For this review, take the finished solid that the model builds, in its own axes (mm). Face numbers are marked on the shaded views. A direction names the side the tool comes from. Give positions to 0.01 mm unless a question says otherwise; leave off trailing zeros. Order: outer loops, then holes, each group sorted by start corner. A loop starts at its lowest first (then second) coordinate and runs counter-clockwise, first axis right, second up. Notation, with made-up numbers: M -38.75,69.25 L -31.75,69.25 A28 cw -31.75,103.25 Z; hole C -1.75,71 d3. An arc over 180 degrees is marked long. Answer as CSV lines item,"result". Start each with the question number.
1. Mouldability with a two-part tool opening along X and no side actions: class the marked faces 1, 2 and 3 as pulls with the +X half, pulls with the -X half, needs draft (parallel to the pull), parting line crosses it, or undercut.
2. We need section D-D, the plane z = 9. Give the boundary of the cut face in (x, y), and give its area (3 significant figures).
3. We need section C-C, the plane x = 7.5. Give the boundary of the cut face in (y, z), and give its area (3 significant figures).
4. Clearance check with flat-ended pins moving along their axes: P1, Ø2.5, axis at x = 7.5, z = 12.5, coming from the +Y side; P2, Ø5, axis at x = 2.5, y = 58, coming from the +Z side. State where each tip first meets the part, or that it passes through.
5. For line 1 along Y through (x, z) = (7.5, 2.8); line 2 along Y through (x, z) = (9.5, 6); line 3 along X through (y, z) = (57.5, 7.25), list the stretches that pass through material, from the lowest coordinate up.
6. Machinability: for the marked faces 4 and 5, which of the approach directions +Z, -Z, +X, -X, +Y, -Y give a long, thin tool a straight path to every point of the face, cutting with its end or side? Answer none if there is none.
7. We need section B-B, the plane z = 12.5. Give the boundary of the cut face in (x, y), and give its area (3 significant figures).
8. We need section A-A, the plane y = 35. Give the boundary of the cut face in (x, z).
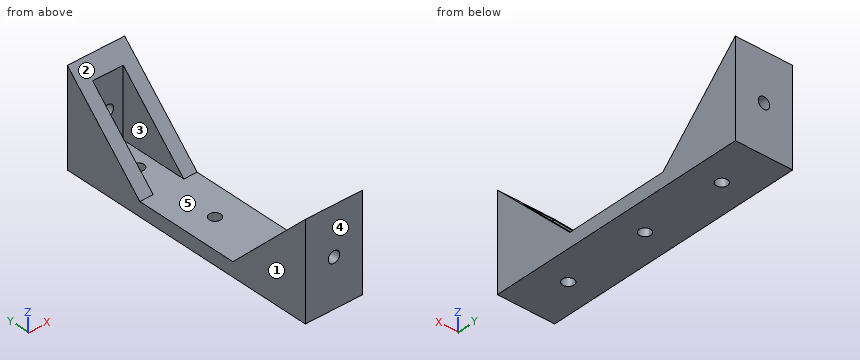
from build123d import *

# Parameters (mm, degrees)
F0_W     = 15
F0_H     = 70
F1_DEPTH = 25
F3_DEPTH = 25
F5_DEPTH = 25
F6_R     = 1.5
F7_DEPTH = 83.8
F8_R     = 1.5
F9_DEPTH = 25


with BuildPart() as f1:
    # F0 (on Top) → F1 (new body)
    with BuildSketch(Plane.XY):
        with Locations((7.5, 35)):
            Rectangle(F0_W, F0_H)
    extrude(amount=F1_DEPTH)

    # F2 (on face) → F3 (cut)
    with BuildSketch(Plane(origin=(0, 0, 0), x_dir=(0, -1, 0), z_dir=(-1, 0, 0))):
        Polygon((-35, 25), (-70, 25), (-48.676951, 3.676951), (-35, 3.676951), (-21.323049, 3.676951), (0, 25), align=None)
    extrude(amount=-F3_DEPTH, mode=Mode.SUBTRACT)

    # F4 (on face) → F5 (cut)
    with BuildSketch(Plane.XY.offset(3.676951)):
        Polygon((3.5, 66.5), (3.5, 35), (3.5, 3.5), (11.5, 3.5), (11.5, 35), (11.5, 66.5), align=None)
    extrude(amount=F5_DEPTH, mode=Mode.SUBTRACT)

    # F6 (on face) → F7 (cut)
    with BuildSketch(Plane.XZ):
        with Locations((7.5, 12.5)):
            Circle(F6_R)
    extrude(amount=-F7_DEPTH, mode=Mode.SUBTRACT)

    # F8 (on face) → F9 (cut)
    with BuildSketch(Plane.XY.offset(3.676951)):
        with Locations((7.5, 57.588476)):
            Circle(F8_R)
        with Locations((7.5, 12.411524)):
            Circle(F8_R)
        with Locations((7.5, 35)):
            Circle(F8_R)
    extrude(amount=-F9_DEPTH, mode=Mode.SUBTRACT)


solid = f1.part
Result set:
1,face 1,"pulls with the -X half"
1,face 2,"needs draft"
1,face 3,"undercut"
2,outline,"M 0,0 L 15,0 L 15,16 L 11.5,16 L 11.5,3.5 L 3.5,3.5 L 3.5,16 L 0,16 Z; M 0,54 L 3.5,54 L 3.5,66.5 L 11.5,66.5 L 11.5,54 L 15,54 L 15,70 L 0,70 Z"
2,area,"280 mm2"
3,outline,"M 0,0 L 10.91,0 L 10.91,3.68 L 3.5,3.68 L 3.5,11 L 0,11 Z; M 0,14 L 3.5,14 L 3.5,21.5 L 0,25 Z; M 13.91,0 L 33.5,0 L 33.5,3.68 L 13.91,3.68 Z; M 36.5,0 L 56.09,0 L 56.09,3.68 L 36.5,3.68 Z; M 59.09,0 L 70,0 L 70,11 L 66.5,11 L 66.5,3.68 L 59.09,3.68 Z; M 66.5,14 L 70,14 L 70,25 L 66.5,21.5 Z"
3,area,"340 mm2"
4,P1,"through"
4,P2,"z = 15.5"
5,line 1,"0 to 10.91, 13.91 to 33.5, 36.5 to 56.09, 59.09 to 70"
5,line 2,"0 to 3.5, 66.5 to 70"
5,line 3,"0 to 3.5, 11.5 to 15"
6,face 4,"+Z, -Z, +X, -X, -Y"
6,face 5,"+Z"
7,outline,"M 0,0 L 6,0 L 6,3.5 L 3.5,3.5 L 3.5,12.5 L 0,12.5 Z; M 0,57.5 L 3.5,57.5 L 3.5,66.5 L 6,66.5 L 6,70 L 0,70 Z; M 9,0 L 15,0 L 15,12.5 L 11.5,12.5 L 11.5,3.5 L 9,3.5 Z; M 9,66.5 L 11.5,66.5 L 11.5,57.5 L 15,57.5 L 15,70 L 9,70 Z"
7,area,"210 mm2"
8,outline,"M 0,0 L 6,0 L 6,3.68 L 0,3.68 Z; M 9,0 L 15,0 L 15,3.68 L 9,3.68 Z"
